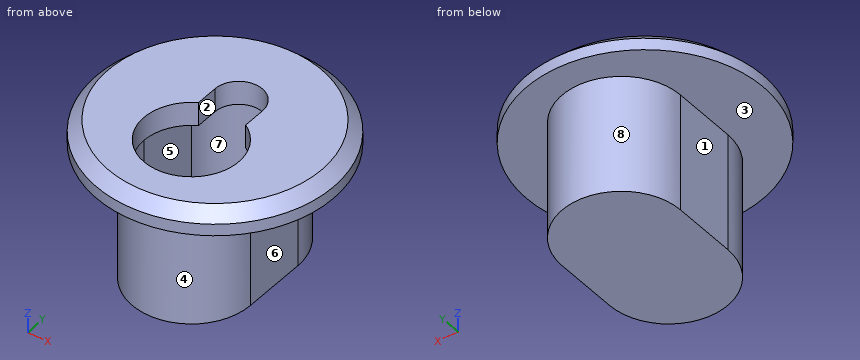
from build123d import *

# Parameters (mm, degrees)
PAD011_DEPTH    = 15
POCKET021_DEPTH = 12
SKETCH036_R     = 15
PAD012_DEPTH    = 3
CHAMFER001_SIZE = 1.5


with BuildPart() as part:
    # Sketch034 → Pad011 (new body)
    with BuildSketch(Plane.XY):
        with BuildLine():
            ThreePointArc((7.5, 8), (0, 15.5), (-7.5, 8))
            Line((-7.5, 8), (-7.5, 0))
            ThreePointArc((-7.5, 0), (0, -7.5), (7.5, 0))
            Line((7.5, 0), (7.5, 8))
        make_face()
    extrude(amount=PAD011_DEPTH)

    # Sketch035 (on Face6 of Pad011) → Pocket021 (cut)
    with BuildSketch(Plane.XY.offset(15)):
        with BuildLine():
            ThreePointArc((-6, 0), (0, -6), (6, 0))
            Line((6, 0), (6, 8))
            ThreePointArc((6, 8), (0, 14), (-6, 8))
            Line((-6, 8), (-6, 0))
        make_face()
    extrude(amount=-POCKET021_DEPTH, mode=Mode.SUBTRACT)

    # Sketch036 (on Face5 of Pocket021) → Pad012 (join)
    with BuildSketch(Plane.XY.offset(15)):
        with Locations((0, 4)):
            Circle(SKETCH036_R)
        with BuildLine():
            ThreePointArc((-3, 5.196152), (0, -6), (3, 5.196152))
            Line((3, 8), (3, 5.196152))
            ThreePointArc((3, 8), (0, 11), (-3, 8))
            Line((-3, 8), (-3, 5.196152))
        make_face(mode=Mode.SUBTRACT)
    extrude(amount=PAD012_DEPTH)

    # Chamfer001
    chamfer001_edges = [part.edges().sort_by_distance(p)[0] for p in [
        (-15, 4, 18),
    ]]
    chamfer(chamfer001_edges, length=CHAMFER001_SIZE)


with BuildPart() as part_1:
    # Body004 placement: moved
    add(part.part.moved(Location((-240, 190, 2))))


solid = part_1.part
Design review of the part built by this model. Coordinates are the model's own, in mm. Face numbers are marked on the shaded views. A direction names the side the tool comes from. Round coordinates to 2 decimals unless told otherwise and drop trailing zeros. Write each loop counter-clockwise with the first axis right and the second up, starting at its lowest first coordinate (ties: lowest second). Pieces come first, ordered by that corner, then holes. Notation, with made-up numbers: (5.5, 22) - (14.5, 22) arc R22 cw to (14.5, 50) - close; hole circle Ø2 at (13.25, 51). An arc over 180 degrees is marked (long way). Use a Markdown table: item, result. Add a question column.
1. Mouldability with a two-part tool opening along Y and no side actions: class the marked faces 6, 7 and 8 as +Y half, -Y half, draft (parallel to the pull), parting line (faces both ways), or undercut.
2. We need section A-A (x = -240). State the section outline as (y, z) points.
3. We need section C-C (y = 194). State the section outline as (x, z) points.
4. For the marked faces 1, 2, 3, 4 and 5, list the 3-axis set-ups (+Z, -Z, +X, -X, +Y, -Y) from which the entire face can be reached by the end or side of a thin tool; tool diameter is ignored.
5. Clearance check with flat-ended pins moving along their axes: pin 1 (9 mm diameter, centred on y = 195.5, z = 7, fed in from +X); pin 2 (2 mm diameter, centred on y = 184, z = 4, fed in from +X); pin 3 (1.4 mm diameter, centred on y = 196, z = 18.5, fed in from -X). State where each tip first meets the part, or that it passes through.
6. We need section B-B (z = 10.5). State the section outline as (x, y) points, then the cut area to 3 significant figures.
7. Wall thickness on probe 1 along Z at (x, y) = (-240, 201.75); probe 2 along X at (y, z) = (194.75, 11.75); probe 3 along Z at (x, y) = (-240.75, 198): over which ranges is each line inside the solid? List them lowest first.
Output:
| question | item | result |
|---|---|---|
| 1 | face 6 | draft |
| 1 | face 7 | undercut |
| 1 | face 8 | +Y half |
| 2 | outline | (179, 17) - (182.5, 17) - (182.5, 2) - (205.5, 2) - (205.5, 17) - (209, 17) - (209, 18.5) - (207.5, 20) - (201, 20) - (201, 17) - (204, 17) - (204, 5) - (184, 5) - (184, 20) - (180.5, 20) - (179, 18.5) - close |
| 3 | outline | (-255, 17) - (-247.5, 17) - (-247.5, 2) - (-232.5, 2) - (-232.5, 17) - (-225, 17) - (-225, 18.5) - (-226.5, 20) - (-235.53, 20) - (-235.53, 17) - (-234, 17) - (-234, 5) - (-246, 5) - (-246, 17) - (-244.47, 17) - (-244.47, 20) - (-253.5, 20) - (-255, 18.5) - close |
| 4 | face 1 | -Z, -X, +Y, -Y |
| 4 | face 2 | +Z |
| 4 | face 3 | -Z |
| 4 | face 4 | -Z, -Y |
| 4 | face 5 | none |
| 5 | pin 1 | stops at x = -232.5 |
| 5 | pin 2 | stops at x = -234.41 |
| 5 | pin 3 | stops at x = -254.94 |
| 6 | outline | (-247.5, 190) arc R7.5 ccw to (-232.5, 190) - (-232.5, 198) arc R7.5 ccw to (-247.5, 198) - close; hole (-246, 190) arc R6 ccw to (-234, 190) - (-234, 198) arc R6 ccw to (-246, 198) - close |
| 6 | area | 87.6 mm2 |
| 7 | probe 1 | z = 2 to 5, 17 to 20 |
| 7 | probe 2 | x = -247.5 to -246, -234 to -232.5 |
| 7 | probe 3 | z = 2 to 5 |
